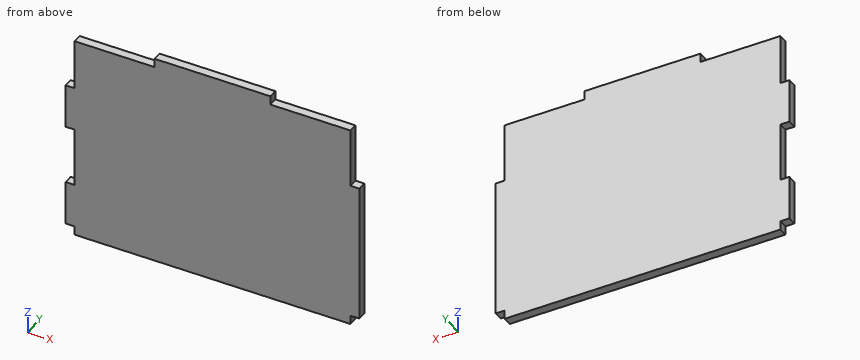
Autodesk Inventor part; units mm, degrees
ref_plane "YZ Plane" through (0, 0, 0) normal (1, 0, 0) x (0, 1, 0)
ref_plane "XZ Plane" through (0, 0, 0) normal (0, 1, 0) x (-1, 0, 0)
ref_plane "XY Plane" through (0, 0, 0) normal (0, 0, 1) x (1, 0, 0)
sketch "Sketch1" plane through (0, 0, 0) normal (0, 1, 0) x (-1, 0, 0)
  point P0 (0, 0)
sketch "Sketch2" plane through (0, 0, 0) normal (0, 1, 0) x (-1, 0, 0)
  line L0 (0, 0) -> (-99, 0)
  line L1 (-99, 0) -> (-99, -90)
  line L2 (-99, -90) -> (0, -90)
  line L3 (0, -90) -> (0, 0)
  dimension "d0" = 99
  dimension "d1" = 90
extrude "Extrusion1" add sketch "Sketch2" along normal blind 3
sketch "Sketch3" plane through (0, 3, 0) normal (0, 1, 0) x (1, 0, 0)
  line L0 (99, 0) -> (99, 90)
  line L1 (99, 0) -> (69, 0)
  line L2 (69, 0) -> (69, 3)
  line L3 (69, 3) -> (99, 3)
  line L4 (99, 3) -> (99, 0)
  line L5 (0, 0) -> (99, 0)
  line L6 (0, 0) -> (30, 0)
  line L7 (30, 0) -> (30, 3)
  line L8 (30, 3) -> (0, 3)
  line L9 (0, 3) -> (0, 0)
  line L10 (0, 3) -> (3, 3)
  line L11 (3, 3) -> (3, 20)
  line L12 (3, 20) -> (0, 20)
  line L13 (0, 20) -> (0, 3)
  line L14 (0, 90) -> (0, 0)
  line L15 (99, 3) -> (96, 3)
  line L16 (96, 3) -> (96, 23)
  line L17 (96, 23) -> (99, 23)
  line L18 (99, 23) -> (99, 3)
  line L19 (99, 90) -> (96, 90)
  line L20 (96, 90) -> (96, 70)
  line L21 (96, 70) -> (99, 70)
  line L22 (99, 70) -> (99, 90)
  line L23 (3, 35) -> (0, 35)
  line L24 (0, 35) -> (0, 55)
  line L25 (0, 55) -> (3, 55)
  line L26 (3, 55) -> (3, 35)
  line L27 (99, 90) -> (0, 90)
  line L28 (0, 90) -> (3, 90)
  line L29 (3, 90) -> (3, 70)
  line L30 (3, 70) -> (0, 70)
  line L31 (0, 70) -> (0, 90)
  dimension "d4" = 30
  dimension "d5" = 3
  dimension "d6" = 30
  dimension "d7" = 3
  dimension "d8" = 3
  dimension "d9" = 17
  dimension "d12" = 3
  dimension "d13" = 20
  dimension "d14" = 3
  dimension "d15" = 20
  dimension "d16" = 20
  dimension "d17" = 3
  dimension "d18" = 15
  dimension "d19" = 3
  dimension "d20" = 15
extrude "Extrusion2" cut sketch "Sketch3" against normal through all contours L1 L2 L3 L0 | L3 L16 L17 L0 | L5 L9 L8 L7 | L21 L20 L19 L0 | L13 L12 L11 L8 | L29 L30 L14 L27 | L14 L25 L26 L23
sketch "Sketch4" plane through (0, 3, 0) normal (0, 1, 0) x (1, 0, 0)
  line L0 (77.6899, 73) -> (37.1359, 73)
  line L1 (69, 3) -> (96, 3)
  line L2 (96, 90) -> (3, 90)
  line L3 (3, 90) -> (3, 70)
  line L4 (96, 90) -> (3, 90)
  line L5 (3, 90) -> (3, 73)
  line L6 (3, 73) -> (96, 73)
  line L7 (96, 73) -> (96, 90)
  point P0 (0, 0)
  dimension "d23" = 70
  dimension "d24" = 70
extrude "Extrusion3" cut sketch "Sketch4" against normal through all
properties part number "top_left_v2"
The listing builds one solid part. Answer for the finished solid, in the listing's coordinates (mm). Coordinates: 2 decimals unless noted, no trailing zeros. Write each loop counter-clockwise with the first axis right and the second up, starting at its lowest first coordinate (ties: lowest second). Pieces come first, ordered by that corner, then holes. Notation, with made-up numbers: (67.5, 41.5) - (102.5, 41.5) arc R13 ccw to (102.5, 63.5) - close; hole circle Ø10 at (-25, 23). An arc over 180 degrees is marked (long way). One line per item, written item: value.
1) Find section C-C (x = 86.5). Give the vertices of the cut face in (y, z).
Geometry check:
outline: (0, -73) - (3, -73) - (3, -3) - (0, -3) - close
2) Find section A-A (y = 1.1). Give the vertices of the cut face in (x, z).
Geometry check:
outline: (0, -70) - (3, -70) - (3, -73) - (96, -73) - (96, -70) - (99, -70) - (99, -23) - (96, -23) - (96, -3) - (69, -3) - (69, 0) - (30, 0) - (30, -3) - (3, -3) - (3, -20) - (0, -20) - (0, -35) - (3, -35) - (3, -55) - (0, -55) - close
3) Consider line 1 along Z through (x, y) = (93.5, 1.8); line 2 along X through (y, z) = (0.9, -46); line 3 along X through (y, z) = (1.95, -22.5). Determine where each line is inside the solid, lowest interval first. Write a range as from..to.
Geometry check:
line 1: z = -73..-3
line 2: x = 3..99
line 3: x = 0..96
4) Each of these flat-tipped pins is pushed along its axis until it touches: pin 1 Ø0.9 at (y, z) = (2, -48.5) entering from -X; pin 2 Ø1.5 at (y, z) = (1, -17) entering from +X; pin 3 Ø0.9 at (x, y) = (97.5, 1.5) entering from +Z. Where does it stop, or does it pass through?
Geometry check:
pin 1: stops at x = 3
pin 2: stops at x = 96
pin 3: stops at z = -23
5) Find section B-B (z = -43). Give the vertices of the cut face in (x, y), and give its area (3 significant figures).
Geometry check:
outline: (3, 0) - (99, 0) - (99, 3) - (3, 3) - close
area: 288 mm2
